Could you check a few things on this model? Use its own coordinates, in mm. A direction names the side the tool comes from. Round coordinates to 2 decimals unless told otherwise and drop trailing zeros. Write each loop counter-clockwise with the first axis right and the second up, starting at its lowest first coordinate (ties: lowest second). Pieces come first, ordered by that corner, then holes. Notation, with made-up numbers: (1.5, 83.25) -> (12.5, 83.25) arc R34 ccw to (12.5, 120.25) -> close; hole circle Ø4 at (89.25, -35.75). An arc over 180 degrees is marked (long way). Answer in a Markdown table with one row per item.
from build123d import *

# Parameters (mm, degrees)
BASPROSKE_W         = 10
BASPROSKE_H         = 9
TOOTHCUT_DEPTH      = 17.186414056
TEETHCUTS_COUNT     = 10
TEETHCUTS_ANGLE     = 324
BORSKE_R            = 2.5
BORE_DEPTH          = 50.0000508
BOSS_EXTRUDE1_DEPTH = 10


with BuildPart() as part:
    # BasProSke → Base-Revolve (revolve)
    with BuildSketch(Plane(origin=(0, 0, 0), x_dir=(1, 0, 0), z_dir=(0, 1, 0)), mode=Mode.PRIVATE) as base_revolve_sk:
        with Locations((5, 4.5)):
            Rectangle(BASPROSKE_W, BASPROSKE_H)
    revolve(base_revolve_sk.sketch.rotate(Axis((-10, 0, 0), (1, 0, 0)), 180), axis=Axis((-10, 0, 0), (1, 0, 0)))

    # TooCutSke → ToothCut (cut, through all)
    with BuildSketch(Plane(origin=(0, 0, 0), x_dir=(0, 0, -1), z_dir=(1, 0, 0))):
        with BuildLine():
            ThreePointArc((0.883878355, 5.554109745), (0, 5.624), (-0.883878355, 5.554109745))
            ThreePointArc((-0.883878355, 5.554109745), (-1.258245767, 7.379188248), (-2.637816971, 8.631324741))
            ThreePointArc((-2.637816971, 8.631324741), (0, 9.0254), (2.637816971, 8.631324741))
            ThreePointArc((2.637816971, 8.631324741), (1.258245767, 7.379188248), (0.883878355, 5.554109745))
        make_face()
    toothcut = extrude(amount=TOOTHCUT_DEPTH, mode=Mode.SUBTRACT)

    # TeethCuts: ToothCut ×10 about axis
    teethcuts_axis = Axis((-10, 0, 0), (1, 0, 0))
    for i in range(1, TEETHCUTS_COUNT):
        add(toothcut.rotate(teethcuts_axis, i * TEETHCUTS_ANGLE / (TEETHCUTS_COUNT - 1)), mode=Mode.SUBTRACT)

    # BorSke → Bore (cut, symmetric)
    with BuildSketch(Plane(origin=(0, 0, 0), x_dir=(0, 0, -1), z_dir=(1, 0, 0))):
        with Locations(Location((0, 0, 0), (0, 0, 180))):
            Circle(BORSKE_R)
    extrude(amount=BORE_DEPTH, both=True, mode=Mode.SUBTRACT)

    # Sketch1 → Boss-Extrude1 (add, through all)
    with BuildSketch(Plane(origin=(10, 0, 0), x_dir=(0, 0, -1), z_dir=(1, 0, 0))):
        with BuildLine():
            Line((0, 2.5), (2.5, 0))
            ThreePointArc((2.5, 0), (1.767766953, 1.767766953), (0, 2.5))
        make_face()
    extrude(amount=-BOSS_EXTRUDE1_DEPTH)


solid = part.part
1) For faces 1 (the face through (4.93, -5.233, 5.362)), 2 (the face through (5.1, 1.3, -1.2)), which set-ups out of +Z, -Z, +X, -X, +Y, -Y let a thin tool reach every point of the face, with its end or its side?
Findings:
| item | result |
|---|---|
| face 1 | +X, -X, -Y |
| face 2 | +X, -X |
2) Imagine slicing it at B-B, the plane z = -1.5. Please give me the cut outline in (x, y).
Findings:
| item | result |
|---|---|
| outline | (0, -7.74) -> (10, -7.74) -> (10, -2) -> (0, -2) -> close; (0, 1) -> (10, 1) -> (10, 7.74) -> (0, 7.74) -> close |
3) Thinking about a two-plate mould opening in Y: for faces 3 (the face through (10, -2, -2)), 4 (the face through (4.93, -4.557, -3.296)), which applies, +Y half, -Y half, draft (parallel to the pull), parting line (faces both ways), or undercut?
Findings:
| item | result |
|---|---|
| face 3 | draft |
| face 4 | undercut |
4) Imagine slicing it at C-C, the plane z = 6. Please give me the cut outline in (x, y).
Findings:
| item | result |
|---|---|
| outline | (0, -5.44) -> (10, -5.44) -> (10, -2.95) -> (0, -2.95) -> close; (0, -1.04) -> (10, -1.04) -> (10, 1.04) -> (0, 1.04) -> close; (0, 2.95) -> (10, 2.95) -> (10, 5.44) -> (0, 5.44) -> close |
5) Please list where these lines run through material, in increasing order: line 1 (Z direction, x = 9.75, y = 5.25); line 2 (Y direction, x = 9.25, z = -6.25); line 3 (Y direction, x = 1.75, z = -1.25).
Findings:
| item | result |
|---|---|
| line 1 | z = -7.31 to -5.4, -2.75 to 2.75, 5.4 to 7.31 |
| line 2 | y = -5.48 to -3.13, -1.1 to 1.1, 3.13 to 5.48 |
| line 3 | y = -7.36 to -2.17, 1.25 to 7.36 |
6) For pin 1 (2 mm diameter, centred on x = 7.5, y = -1.5, fed in from +Z); pin 2 (6 mm diameter, centred on x = 6, y = 5.5, fed in from -Z), each with a flat end and sliding along its axis, tell me the tip position at first contact or that it passes through.
Findings:
| item | result |
|---|---|
| pin 1 | stops at z = 8.66 |
| pin 2 | stops at z = -7.39 |
7) Imagine slicing it at A-A, the plane y = -6.75. Please give me the cut outline in (x, z), plus the area to 3 significant figures.
Findings:
| item | result |
|---|---|
| outline | (0, -3.32) -> (10, -3.32) -> (10, -0.99) -> (0, -0.99) -> close; (0, 0.99) -> (10, 0.99) -> (10, 3.32) -> (0, 3.32) -> close |
| area | 46.7 mm^2 |
